Geometry: final body of the model. Coordinates: model frame, mm. A direction names the side the tool comes from. Coordinates: 2 decimals unless noted, no trailing zeros. Loops run counter-clockwise (first coordinate to the right, second up) from the corner with the lowest first, then second, coordinate; pieces in that order, holes last. Notation, with made-up numbers: (-5, -21.75) - (18, -21.75) arc R11 cw to (18, -7.75) - close; hole circle Ø11 at (-10, 2.25). An arc over 180 degrees is marked (long way). Put each result on its own line as item: value. Start each with the question number.
1) Contact query for flat-ended pins moving along their axis: pin 1 Ø2 at (y, z) = (1, -10.5) entering from +X; pin 2 Ø2.5 at (x, z) = (-6.59, 4.52) entering from +Y; pin 3 Ø13 at (x, z) = (-10.5, -6.5) entering from +Y. Output: stop coordinate, or through.
2) Section B-B on y = 2. Output: boundary loops of the cut face in (x, z).
3) Section C-C on x = -18. Output: boundary loops of the cut face in (y, z), and give its area (3 significant figures).
4) Draft query along Y for faces 1 (the flat face through (-19, 2, 22.019)), 2 (the cylindrical face through (-22.89, 5.92, 4.2)), 3 (the cylindrical face through (-4.178, 0.035, -13.395)). Return one class per face: +Y half, -Y half, draft (parallel to the pull), parting line (faces both ways), or undercut.
5) Material intervals for line 1 along Y through (x, z) = (0, -1.5); line 2 along X through (y, z) = (2.75, 10.5); line 3 along Z through (x, y) = (-21.25, 4.75), sorted ascending. Write a range as from..to.
6) Section D-D on y = -0.5. Output: boundary loops of the cut face in (x, z), and give its area (3 significant figures).
7) Reachability of faces 4 (the cylindrical face through (-3.927, 0.035, 22.193)), 5 (the cylindrical face through (-9.574, 4.965, 2.616)), 6 (the cylindrical face through (-23.29, 2.32, 2.25)), 7 (the flat face through (-19, 3, 27.019)), 8 (the flat face through (-22.2, 5.5, -17.981)) from +Z, -Z, +X, -X, +Y, -Y: full face, straight path, thin tool, end or side. Return the list, or none.
8) Section A-A on z = 0.5. Output: boundary loops of the cut face in (x, y).
```python
from build123d import *
from build123d.topology import SkipClean

# Parameters (mm, degrees)
BOSS_EXTRUDE7_DEPTH      = 2.5
BOSS_EXTRUDE7_DEPTH_BACK = 2.5
SKETCH1_R                = 1
SKETCH3_W                = 5
SKETCH3_H                = 5
SKETCH3_R                = 1
BOSS_EXTRUDE9_DEPTH      = 1
FILLET2_R                = 2.5
SKETCH4_R                = 3.54
SKETCH4_R_2              = 2.5
BOSS_EXTRUDE11_DEPTH     = 5
BOSS_EXTRUDE13_START     = -4
BOSS_EXTRUDE13_DEPTH     = 4
CIRPATTERN2_COUNT        = 21
SKETCH18_R               = 5
SKETCH18_R_2             = 4.05
BOSS_EXTRUDE24_DEPTH     = 45
SKETCH19_R               = 4.05
CUT_EXTRUDE2_DEPTH       = 55.105925545
BOSS_EXTRUDE25_START     = -5
SKETCH20_R               = 5
BOSS_EXTRUDE25_DEPTH     = 5
CUT_EXTRUDE4_DEPTH       = 45
BOSS_EXTRUDE35_DEPTH     = 5
SKETCH28_W               = 5
SKETCH28_H               = 1.900081374
CUT_EXTRUDE9_DEPTH       = 45
CUT_EXTRUDE10_DEPTH      = 45
CUT_EXTRUDE12_DEPTH      = 40
CUT_EXTRUDE12_DEPTH_BACK = 40
SKETCH32_R               = 4.05
CUT_EXTRUDE13_START      = -40
SKETCH33_R               = 1
CUT_EXTRUDE13_DEPTH      = 40


with BuildPart() as part:
    # Sketch1 → Boss-Extrude7 (new, two sides: drawn at the far end of the back side and taken through both)
    with BuildSketch(Plane(origin=(0, 0, 0), x_dir=(1, 0, 0), z_dir=(0, 1, 0)).offset(-BOSS_EXTRUDE7_DEPTH_BACK)):
        Polygon((-29.089537279, -2.019014343), (-29.089537279, -7.019014343), (-14.392838138, -12.322315202), (-9.089537279, -27.019014343), (-4.089537279, -27.019014343), (1.21376358, -12.322315202), (15.910462721, -7.019014343), (15.910462721, -2.019014343), (1.21376358, 3.284286516), (-4.089537279, 17.980985657), (-9.089537279, 17.980985657), (-14.392838138, 3.284286516), align=None)
        with Locations(Location((-6.589537279, -4.519014343, 0), (0, 0, 270))):
            Circle(SKETCH1_R, mode=Mode.SUBTRACT)
    extrude(amount=BOSS_EXTRUDE7_DEPTH + BOSS_EXTRUDE7_DEPTH_BACK)

    # Sketch3 → Boss-Extrude9 (add)
    with BuildSketch(Plane(origin=(0, 2.5, 0), x_dir=(1, 0, 0), z_dir=(0, 1, 0))):
        with Locations((-6.589537279, -4.519014343)):
            Rectangle(SKETCH3_W, SKETCH3_H)
        with Locations(Location((-6.589537279, -4.519014343, 0), (0, 0, 270))):
            Circle(SKETCH3_R, mode=Mode.SUBTRACT)
    extrude(amount=BOSS_EXTRUDE9_DEPTH)

    # Fillet2
    fillet2_edges = [part.edges().sort_by_distance(p)[0] for p in [
        (-4.089537279, 3, 7.019014343),
        (-4.089537279, 3, 2.019014343),
        (-9.089537279, 3, 7.019014343),
        (-9.089537279, 3, 2.019014343),
    ]]
    fillet(fillet2_edges, radius=FILLET2_R - 0.0001)  # a hair under: the kernel refuses the full size

    # Sketch4 → Boss-Extrude11 (add)
    with BuildSketch(Plane(origin=(0, 2.5, 0), x_dir=(1, 0, 0), z_dir=(0, 1, 0))):
        with Locations(Location((-6.589537279, -4.519014343, 0), (0, 0, 90))):
            Circle(SKETCH4_R)
        with Locations(Location((-6.589537279, -4.519014343, 0), (0, 0, 90))):
            Circle(SKETCH4_R_2, mode=Mode.SUBTRACT)
    extrude(amount=BOSS_EXTRUDE11_DEPTH)

    # Sketch8 → Boss-Extrude13 (add)
    with BuildSketch(Plane(origin=(0, 7.5, 0), x_dir=(1, 0, 0), z_dir=(0, 1, 0)).offset(BOSS_EXTRUDE13_START)):
        with BuildLine():
            ThreePointArc((-7.641010895, -2.250886649), (-7.405163574, -2.347475501), (-7.291219912, -2.119505751))
            ThreePointArc((-7.291219912, -2.119505751), (-7.468573367, -2.178652072), (-7.641010895, -2.250886649))
        make_face()
    boss_extrude13 = extrude(amount=BOSS_EXTRUDE13_DEPTH)

    # CirPattern2: Boss-Extrude13 ×21 about axis
    cirpattern2_axis = Axis((-6.589537279, 0, 4.519014343), (0, 1, 0))
    for i in range(1, CIRPATTERN2_COUNT):
        add(boss_extrude13.rotate(cirpattern2_axis, i * 360 / CIRPATTERN2_COUNT))

    # Sketch18 → Boss-Extrude24 (add)
    with BuildSketch(Plane(origin=(0, 0, -17.980985657), x_dir=(-1, 0, 0), z_dir=(0, 0, -1))):
        with Locations((19.242838138, 2.5)):
            Circle(SKETCH18_R)
        with Locations((19.242838138, 2.5)):
            Circle(SKETCH18_R_2, mode=Mode.SUBTRACT)
    extrude(amount=-BOSS_EXTRUDE24_DEPTH)

    # Sketch19 → Cut-Extrude2 (cut, through all)
    with BuildSketch(Plane(origin=(0, 0, -17.980985657), x_dir=(-1, 0, 0), z_dir=(0, 0, -1))):
        with Locations((19.242838138, 2.5)):
            Circle(SKETCH19_R)
    extrude(amount=-CUT_EXTRUDE2_DEPTH, mode=Mode.SUBTRACT)

    # Sketch20 → Boss-Extrude25 (add)
    with BuildSketch(Plane.XY.offset(27.019014343).offset(BOSS_EXTRUDE25_START)):
        with Locations(Location((-19.242838138, 2.5, 0), (0, 0, 180))):
            Circle(SKETCH20_R)
    extrude(amount=BOSS_EXTRUDE25_DEPTH)

    # Sketch24 → Cut-Extrude4 (cut)
    with SkipClean():  # the faces are left unmerged after this step: merging them gives an invalid solid
        with BuildSketch(Plane(origin=(0, 0, -17.980985657), x_dir=(-1, 0, 0), z_dir=(0, 0, -1))):
            with BuildLine():
                Line((19.242838138, -2.5), (29.239649505, -2.5))
                Line((29.239649505, -2.5), (29.239649505, 2.5))
                Line((29.239649505, 2.5), (24.242838138, 2.5))
                ThreePointArc((24.242838138, 2.5), (22.778372044, -1.035533906), (19.242838138, -2.5))
            make_face()
        extrude(amount=-CUT_EXTRUDE4_DEPTH, mode=Mode.SUBTRACT)

    # Sketch26 → Boss-Extrude35 (add)
    with BuildSketch(Plane(origin=(0, 2.5, 0), x_dir=(1, 0, 0), z_dir=(0, 1, 0))):
        with BuildLine():
            Line((1.21376358, 3.284286516), (1.21376358, -12.322315202))
            ThreePointArc((1.21376358, -12.322315202), (-5.970751226, -23.907365708), (-19.242838138, -27.019014343))
            Line((-19.242838138, -27.019014343), (-19.242838138, 17.980985657))
            ThreePointArc((-19.242838138, 17.980985657), (-5.970751226, 14.869337023), (1.21376358, 3.284286516))
        make_face()
    extrude(amount=-BOSS_EXTRUDE35_DEPTH)

    # Sketch28 → Cut-Extrude9 (cut)
    with BuildSketch(Plane(origin=(0, 2.5, 0), x_dir=(1, 0, 0), z_dir=(0, 1, 0))):
        Polygon((-19.242838138, 17.980985657), (-14.291903713, 18.094552541), (-14.291903713, 20.179520428), (-19.242838138, 20.179520428), align=None)
        with Locations((-16.742838138, -27.96905503)):
            Rectangle(SKETCH28_W, SKETCH28_H)
    extrude(amount=-CUT_EXTRUDE9_DEPTH, mode=Mode.SUBTRACT)

    # Sketch30 → Cut-Extrude10 (cut)
    with BuildSketch(Plane(origin=(0, 2.5, 0), x_dir=(1, 0, 0), z_dir=(0, 1, 0))):
        with BuildLine():
            Line((1.21376358, 3.284286516), (1.21376358, -12.322315202))
            ThreePointArc((1.21376358, -12.322315202), (-5.970751226, -23.907365708), (-19.242838138, -27.019014343))
            Line((-19.242838138, -27.019014343), (-19.242838138, -29.875538086))
            Line((-19.242838138, -29.875538086), (19.285813169, -29.875538086))
            Line((19.285813169, -29.875538086), (19.285813169, 19.780165104))
            Line((19.285813169, 19.780165104), (-19.242838138, 19.780165104))
            Line((-19.242838138, 19.780165104), (-19.242838138, 17.980985657))
            ThreePointArc((-19.242838138, 17.980985657), (-5.970751226, 14.869337023), (1.21376358, 3.284286516))
        make_face()
    extrude(amount=-CUT_EXTRUDE10_DEPTH, mode=Mode.SUBTRACT)

    # Sketch32 → Cut-Extrude12 (cut, two sides: drawn at the far end of the back side and taken through both)
    with BuildSketch(Plane(origin=(0, 0, -17.980985657), x_dir=(-1, 0, 0), z_dir=(0, 0, -1)).offset(-CUT_EXTRUDE12_DEPTH_BACK)):
        with Locations(Location((19.242838138, 2.5, 0), (0, 0, 180))):
            Circle(SKETCH32_R)
    extrude(amount=CUT_EXTRUDE12_DEPTH + CUT_EXTRUDE12_DEPTH_BACK, mode=Mode.SUBTRACT)

    # Sketch33 → Cut-Extrude13 (cut)
    with BuildSketch(Plane(origin=(0, 2.5, 0), x_dir=(1, 0, 0), z_dir=(0, 1, 0)).offset(CUT_EXTRUDE13_START)):
        with Locations(Location((-6.589537279, -4.519014343, 0), (0, 0, 270))):
            Circle(SKETCH33_R)
    extrude(amount=CUT_EXTRUDE13_DEPTH, mode=Mode.SUBTRACT)


solid = part.part
```
Answer block:
1. pin 1: stops at x = -1.05
1. pin 2: stops at y = 3.5
1. pin 3: stops at y = 6.97
2. outline: (-24.22, -17.98) - (-23.26, -17.98) - (-23.26, 22.02) - (-15.22, 22.02) - (-15.22, -18.07) - (-14.29, -18.09) arc R17.81 ccw to (1.21, -3.28) - (1.21, 12.32) arc R17.81 ccw to (-14.24, 27.13) - (-14.24, 27.02) - (-24.22, 27.02) - close; hole circle Ø2 at (-6.59, 4.52)
3. outline: (-2.5, -18.01) - (-1.35, -18.01) - (-1.35, 22.02) - (6.35, 22.02) - (6.35, -17.98) - (7.34, -17.98) - (7.34, 27.02) - (-2.5, 27.02) - close
3. area: 135 mm²
4. face 1: undercut
4. face 2: parting line
4. face 3: draft
5. line 1: y = -2.5..2.5
5. line 2: x = -24.24..-23.29, -15.2..-14.25
5. line 3: z = 22.02..27.02
6. outline: (-23.24, -17.98) - (-21.96, -17.98) - (-21.96, 22.02) - (-16.52, 22.02) - (-16.52, -18.04) - (-14.29, -18.09) arc R17.81 ccw to (1.21, -3.28) - (1.21, 12.32) arc R17.81 ccw to (-14.24, 27.13) - (-14.24, 27.02) - (-23.24, 27.02) - close; hole circle Ø2 at (-6.59, 4.52)
6. area: 759 mm²
7. face 4: +Z, +X, +Y, -Y
7. face 5: +Y
7. face 6: -Z
7. face 7: +Z, -X, +Y, -Y
7. face 8: -Z, -X, +Y
8. outline: (-19.24, -2.5) - (1.21, -2.5) - (1.21, 2.5) - (-14.24, 2.5) arc R5 ccw (long way) to start; hole circle Ø8.1 at (-19.24, 2.5)
